```python
from build123d import *

# Parameters (mm, degrees)
F0_W     = 355.6
F0_H     = 355.6
F1_DEPTH = 6.35
F2_R     = 2.5
F2_W     = 25.4
F2_H     = 68.58
F3_DEPTH = 6.351
F4_DEPTH = 6.351
F5_DEPTH = 6.351


with BuildPart() as f1:
    # F0 (on Top) → F1 (new body)
    with BuildSketch(Plane.XY):
        with Locations((-134.099856, -1.412397)):
            Rectangle(F0_W, F0_H)
    extrude(amount=F1_DEPTH)

    # F2 (on face) → F3 (cut, through all)
    with BuildSketch(Plane.XY.offset(6.35)):
        with Locations((-286.499856, 163.687603)):
            Circle(F2_R)
        with Locations((-286.499856, -166.512397)):
            Circle(F2_R)
        with Locations((18.300144, -166.512397)):
            Circle(F2_R)
        with Locations((18.300144, 163.687603)):
            Circle(F2_R)
        with Locations((-286.499856, -124.145197)):
            Circle(F2_R)
        with Locations((-286.499856, 121.320403)):
            Circle(F2_R)
        with Locations((18.300144, 121.320403)):
            Circle(F2_R)
        with Locations((18.300144, -124.145197)):
            Circle(F2_R)
        with Locations((-261.099856, 129.397603)):
            Rectangle(F2_W, F2_H)
    extrude(amount=-F3_DEPTH, mode=Mode.SUBTRACT)

    # F2 (on face) → F4 (cut, through all)
    with BuildSketch(Plane.XY.offset(6.35)):
        with Locations((-286.499856, 163.687603)):
            Circle(F2_R)
        with Locations((-286.499856, -166.512397)):
            Circle(F2_R)
        with Locations((18.300144, -166.512397)):
            Circle(F2_R)
        with Locations((18.300144, 163.687603)):
            Circle(F2_R)
        with Locations((-286.499856, -124.145197)):
            Circle(F2_R)
        with Locations((-286.499856, 121.320403)):
            Circle(F2_R)
        with Locations((18.300144, 121.320403)):
            Circle(F2_R)
        with Locations((18.300144, -124.145197)):
            Circle(F2_R)
        with Locations((-261.099856, 129.397603)):
            Rectangle(F2_W, F2_H)
    extrude(amount=-F4_DEPTH, mode=Mode.SUBTRACT)

    # F2 (on face) → F5 (cut, through all)
    with BuildSketch(Plane.XY.offset(6.35)):
        with Locations((-286.499856, 163.687603)):
            Circle(F2_R)
        with Locations((-286.499856, -166.512397)):
            Circle(F2_R)
        with Locations((18.300144, -166.512397)):
            Circle(F2_R)
        with Locations((18.300144, 163.687603)):
            Circle(F2_R)
        with Locations((-286.499856, -124.145197)):
            Circle(F2_R)
        with Locations((-286.499856, 121.320403)):
            Circle(F2_R)
        with Locations((18.300144, 121.320403)):
            Circle(F2_R)
        with Locations((18.300144, -124.145197)):
            Circle(F2_R)
    extrude(amount=-F5_DEPTH, mode=Mode.SUBTRACT)


solid = f1.part
```
Geometry: final body of the model. Coordinates: model frame, mm. Coordinates: 2 decimals unless noted, no trailing zeros. Loops run counter-clockwise (first coordinate to the right, second up) from the corner with the lowest first, then second, coordinate; pieces in that order, holes last. Notation, with made-up numbers: (-3.75, 70.5) -> (11.25, 70.5) arc R15 cw to (11.25, 84.5) -> close; hole circle Ø9 at (9, 2.25). An arc over 180 degrees is marked (long way). Use a Markdown table: item, result. Add a question column.
(1) Section query A-A, the plane y = 142. Return loops of the section in (x, z).
(2) Line query: line 1 along Y through (x, z) = (19.5, 1.25); line 2 along X through (y, z) = (103, 4.75); line 3 along Y through (x, z) = (-265.5, 3). Output: solid intervals per line, ascending.
(3) Section query B-B, the plane z = 1.75. State how many separate pieces and enclosed holes the cut face has, plus the area to 3 significant figures.
Answer:
| question | item | result |
|---|---|---|
| 1 | outline | (-311.9, 0) -> (-273.8, 0) -> (-273.8, 6.35) -> (-311.9, 6.35) -> close; (-248.4, 0) -> (43.7, 0) -> (43.7, 6.35) -> (-248.4, 6.35) -> close |
| 2 | line 1 | y = -179.21 to -168.71, -164.32 to -126.34, -121.95 to 119.13, 123.51 to 161.49, 165.88 to 176.39 |
| 2 | line 2 | x = -311.9 to -273.8, -248.4 to 43.7 |
| 2 | line 3 | y = -179.21 to 95.11, 163.69 to 176.39 |
| 3 | separate pieces | 1 |
| 3 | enclosed holes | 9 |
| 3 | area | 125,000 mm^2 |
